Model file for the job. Use its own axes, mm. Give positions to 0.01 mm unless a question says otherwise; leave off trailing zeros. Loops run counter-clockwise (first coordinate to the right, second up) from the corner with the lowest first, then second, coordinate; pieces in that order, holes last. Notation, with made-up numbers: M 48.25,-38.5 L 81.25,-38.5 A10 cw 81.25,-19.5 Z; hole C 6,43.25 d8. An arc over 180 degrees is marked long. Use CSV: the item, a comma, the result in double quotes. Start each with the question number.
(1) Wall check: line 1 along X through (y, z) = (19.75, 0); line 2 along Z through (x, y) = (279.4, 12.75); line 3 along X through (y, z) = (23, -2). Give the ranges that are in metal, low to high. Write a range as from..to.
(2) Slice it at A-A on x = -139.7. List the corners of the cut face in (y, z).
(3) Slice it at B-B on z = 0. List the corners of the cut face in (x, y).
Autodesk Inventor part; units mm, degrees
ref_plane "YZ Plane" through (0, 0, 0) normal (1, 0, 0) x (0, 1, 0)
ref_plane "XZ Plane" through (0, 0, 0) normal (0, 1, 0) x (-1, 0, 0)
ref_plane "XY Plane" through (0, 0, 0) normal (0, 0, 1) x (1, 0, 0)
sketch "Sketch1" plane through (0, 0, 0) normal (0, 1, 0) x (-1, 0, 0)
  line L0 (304.8, 38.1) -> (-304.8, 38.1)
  line L1 (-304.8, 38.1) -> (-304.8, -38.1)
  line L2 (-304.8, -38.1) -> (304.8, -38.1)
  line L3 (304.8, -38.1) -> (304.8, 38.1)
  line L4 (304.8, 38.1) -> (-304.8, -38.1) construction
  line L5 (-304.8, 38.1) -> (304.8, -38.1) construction
  point P0 (0, 0)
  dimension "d0" = 609.6
  dimension "d1" = 76.2
extrude "Extrusion1" add sketch "Sketch1" along normal blind 25.4
sketch "Sketch2" plane through (0, 25.4, 0) normal (0, 1, 0) x (1, 0, 0)
  line L0 (0, 0) -> (0, 46.0964) construction
  line L1 (0, 0) -> (279.4, 0) construction
  line L2 (0, 0) -> (139.7, 0) construction
  point P0 (-139.7, 0)
  point P1 (-279.4, 0)
  dimension "d4" = 279.4
  dimension "d5" = 139.7
hole "Hole1" at (139.7, 25.4, 0) at (279.4, 25.4, 0) at (-139.7, 25.4, 0) at (-279.4, 25.4, 0) direction (0, -1, 0) diameter 10.0838 end through all
sketch "Sketch3" plane through (0, 25.4, 0) normal (0, 1, 0) x (1, 0, 0)
  line L0 (7.3025, 18.161) -> (-7.3025, 18.161) construction
  line L1 (-7.3025, 18.161) -> (-7.3025, -18.161) construction
  line L2 (-7.3025, -18.161) -> (7.3025, -18.161) construction
  line L3 (7.3025, -18.161) -> (7.3025, 18.161) construction
  line L4 (7.3025, 18.161) -> (-7.3025, -18.161) construction
  line L5 (-7.3025, 18.161) -> (7.3025, -18.161) construction
  point P0 (0, 0)
  dimension "d13" = 14.605
  dimension "d14" = 36.322
hole "Hole2" at (-7.3025, 25.4, -18.161) at (7.3025, 25.4, -18.161) at (7.3025, 25.4, 18.161) at (-7.3025, 25.4, 18.161) direction (0, -1, 0) diameter 3.9624 end through all
properties part number "table reinforcement"
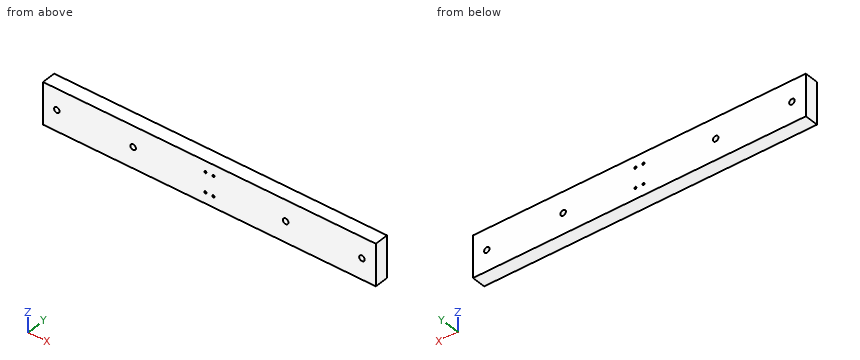
Reply:
1,line 1,"x = -304.8..-284.44, -274.36..-144.74, -134.66..134.66, 144.74..274.36, 284.44..304.8"
1,line 2,"z = -38.1..-5.04, 5.04..38.1"
1,line 3,"x = -304.8..-284.03, -274.77..-144.33, -135.07..135.07, 144.33..274.77, 284.03..304.8"
2,outline,"M 0,-38.1 L 25.4,-38.1 L 25.4,-5.04 L 0,-5.04 Z; M 0,5.04 L 25.4,5.04 L 25.4,38.1 L 0,38.1 Z"
3,outline,"M -304.8,0 L -284.44,0 L -284.44,25.4 L -304.8,25.4 Z; M -274.36,0 L -144.74,0 L -144.74,25.4 L -274.36,25.4 Z; M -134.66,0 L 134.66,0 L 134.66,25.4 L -134.66,25.4 Z; M 144.74,0 L 274.36,0 L 274.36,25.4 L 144.74,25.4 Z; M 284.44,0 L 304.8,0 L 304.8,25.4 L 284.44,25.4 Z"
